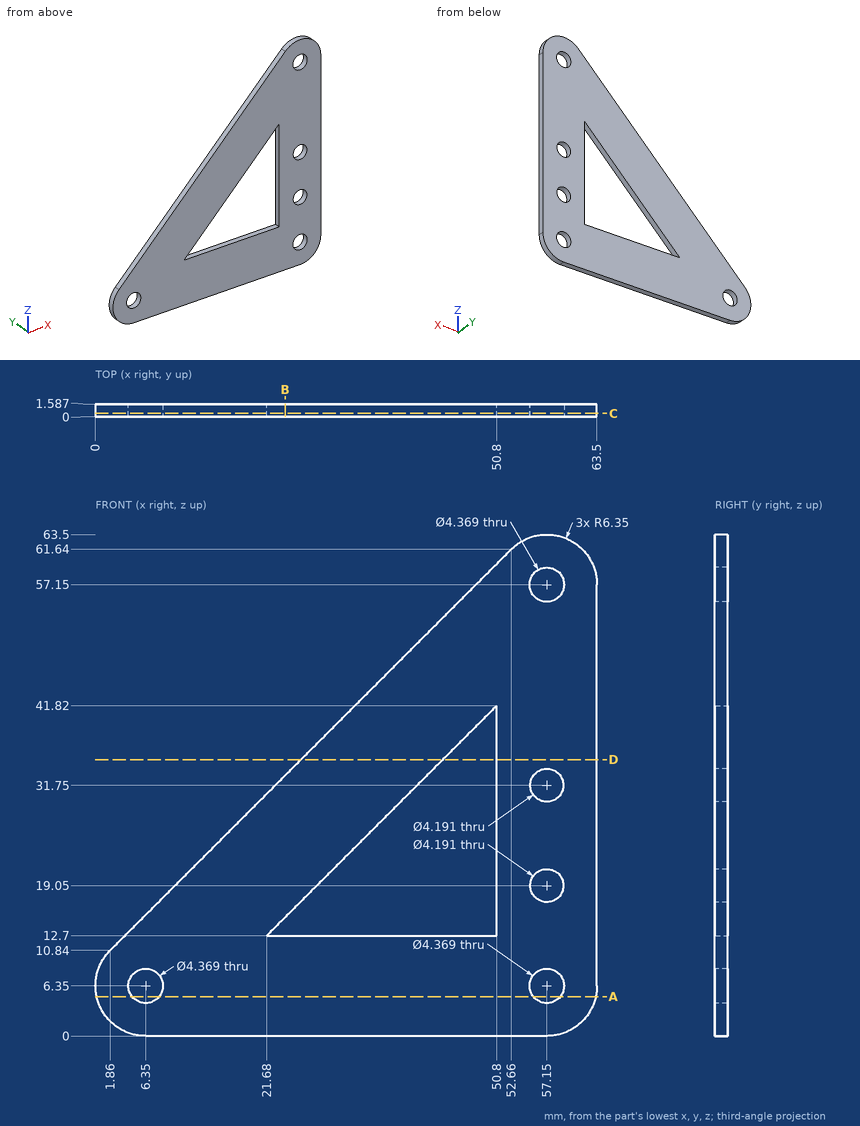
Design review of the part shown in the three views and the two pictorial views. Dimensions are in mm from the part's minimum x, y and z. Give positions to 0.01 mm unless a question says otherwise; leave off trailing zeros. Loops run counter-clockwise (first coordinate to the right, second up) from the corner with the lowest first, then second, coordinate; pieces in that order, holes last. Notation, with made-up numbers: M 77.25,-38 L 86.25,-38 A10 cw 86.25,-34 Z; hole C 12.5,-10 d3. An arc over 180 degrees is marked long. Write item = value, one per line.
Q1. We need section A-A (z = 5). Give the boundary of the cut face in (x, y) (1 decimal).
Output values:
outline = M 0.1,0 L 4.6,0 L 4.6,1.6 L 0.1,1.6 Z; M 8.1,0 L 55.4,0 L 55.4,1.6 L 8.1,1.6 Z; M 58.9,0 L 63.4,0 L 63.4,1.6 L 58.9,1.6 Z
Q2. Insertion check: pin 1 (0.5 mm diameter, centred on y = 0.5, z = 23.5, fed in from -X). The pin has a flat end and moves straight along its axis. Give the tip position at first contact, or say it passes through.
Output values:
pin_1 = 14.27
Q3. We need section D-D (z = 35). Give the boundary of the cut face in (x, y).
Output values:
outline = M 26.02,0 L 43.98,0 L 43.98,1.59 L 26.02,1.59 Z; M 50.8,0 L 63.5,0 L 63.5,1.59 L 50.8,1.59 Z
Q4. We need section C-C (y = 0.4). Count the separate pieces of the cut face and the enclosed holes in it, plus the area to 3 significant figures.
Output values:
separate_pieces = 1
enclosed_holes = 6
area = 2,020 mm^2
Q5. We need section B-B (x = 24). Give the boundary of the cut face in (y, z).
Output values:
outline = M 0,0 L 1.59,0 L 1.59,12.7 L 0,12.7 Z; M 0,15.02 L 1.59,15.02 L 1.59,32.98 L 0,32.98 Z
Q6. To check wall thickness, follow line 1 (Z direction, x = 57.5, y = 1) (1 decimal); line 2 (X direction, y = 0.6, z = 18) (1 decimal); line 3 (X direction, y = 1.55, z = 56) (1 decimal). State the ranges of each line that lie inside material, in increasing order. Write a range as [from, to].
Output values:
line_1 = [0, 4.2], [8.5, 17], [21.1, 29.7], [33.8, 55], [59.3, 63.5]
line_2 = [9, 27], [50.8, 55.3], [59, 63.5]
line_3 = [47, 55.3], [59, 63.5]
